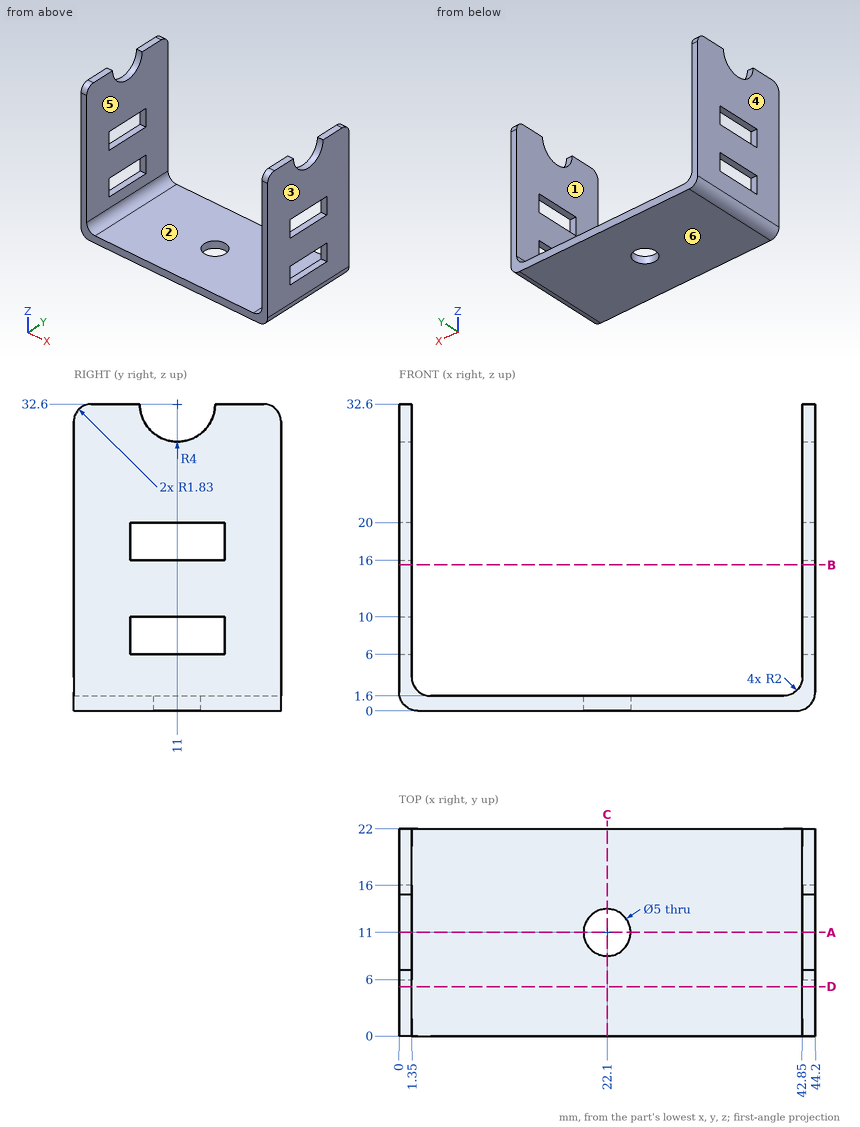
Could you check a few things on this drawing? It's one solid part, dimensions in mm from its lowest x, y, z. A direction names the side the tool comes from. Round coordinates to 2 decimals unless told otherwise and drop trailing zeros. Order: outer loops, then holes, each group sorted by start corner. A loop starts at its lowest first (then second) coordinate and runs counter-clockwise, first axis right, second up.
Q1. Please list where these lines run through material, in increasing order: probe 1 along X at (y, z) = (19.25, 6); probe 2 along Y at (x, z) = (22.1, 1); probe 3 along Z at (x, y) = (40, 13.75).
Geometry says:
probe 1: x = 0 to 1.35, 42.85 to 44.2
probe 2: y = 0 to 8.5, 13.5 to 22
probe 3: z = 0 to 1.6
Q2. Imagine slicing it at B-B, the plane z = 15.5. List the corners of the cut face in (x, y) for me.
Geometry says:
outline: (0, 0) - (1.35, 0) - (1.35, 22) - (0, 22) - close; (42.85, 0) - (44.2, 0) - (44.2, 22) - (42.85, 22) - close
Q3. Imagine slicing it at C-C, the plane x = 22.1. List the corners of the cut face in (y, z) for me, then the cut area to 3 significant figures.
Geometry says:
outline: (0, 0) - (8.5, 0) - (8.5, 1.6) - (0, 1.6) - close; (13.5, 0) - (22, 0) - (22, 1.6) - (13.5, 1.6) - close
area: 27.2 mm2
Q4. Which directions (+Z, -Z, +X, -X, +Y, -Y) give clear straight access to the entire face, cutting with the end or side of a thin tool? Please do the marked faces 5 and 6.
Geometry says:
face 5: +Z, +Y, -Y
face 6: -Z, +X, -X, +Y, -Y
Q5. Imagine slicing it at D-D, the plane y = 5.25. List the corners of the cut face in (x, z) for me.
Geometry says:
outline: (0, 2) arc R2 ccw to (2, 0) - (42.2, 0) arc R2 ccw to (44.2, 2) - (44.2, 32.6) - (42.85, 32.6) - (42.85, 3.6) arc R2 cw to (40.85, 1.6) - (3.35, 1.6) arc R2 cw to (1.35, 3.6) - (1.35, 32.6) - (0, 32.6) - close
Q6. Imagine slicing it at A-A, the plane y = 11. State how many separate pieces and enclosed holes the cut face has, then the cut area to 3 significant figures.
Geometry says:
separate pieces: 6
enclosed holes: 0
area: 114 mm2
Q7. I'm going to push flat-ended pins straight in: P1, Ø1.1, axis at x = 44, y = 12.5, coming from the -Z side; P2, Ø2, axis at x = 31, y = 13, coming from the +Z side; P3, Ø1.5, axis at x = 1, y = 10, coming from the +Z side. Where does each tip first touch, or does it pass through?
Geometry says:
P1: stops at z = 0.44
P2: stops at z = 1.6
P3: stops at z = 29
Q8. Thinking about a two-plate mould opening in X: for the marked faces 1, 2, 3 and 4, which applies, released by +X, released by -X, zero draft, split by the parting line, or undercut?
Geometry says:
face 1: undercut
face 2: undercut
face 3: released by +X
face 4: released by -X
